```python
from build123d import *

# Parameters (mm, degrees)
SKETCH1_R           = 30
SKETCH1_R_2         = 7
BOSS_EXTRUDE1_DEPTH = 10
CUT_EXTRUDE1_DEPTH  = 161.838428244


with BuildPart() as part:
    # Sketch1 → Boss-Extrude1 (new, symmetric)
    with BuildSketch(Plane.XY):
        with BuildLine():
            Line((27.935473676, -25.760615491), (128.063755469, -9.084385863))
            ThreePointArc((128.063755469, -9.084385863), (155, 0), (128.063755469, 9.084385863))
            Line((128.063755469, 9.084385863), (27.935473676, 25.760615491))
            ThreePointArc((27.935473676, 25.760615491), (-38, 0), (27.935473676, -25.760615491))
        make_face()
        Circle(SKETCH1_R, mode=Mode.SUBTRACT)
        with Locations((140, 0)):
            Circle(SKETCH1_R_2, mode=Mode.SUBTRACT)
    extrude(amount=BOSS_EXTRUDE1_DEPTH, both=True)

    # Sketch2 → Cut-Extrude1 (cut, through all)
    with BuildSketch(Plane.XY.offset(10)):
        with BuildLine():
            Line((46.591424383, 15.557071672), (100.514303988, 6.576289156))
            ThreePointArc((100.514303988, 6.576289156), (106.085905266, 0), (100.514303988, -6.576289156))
            Line((100.514303988, -6.576289156), (46.591424383, -15.557071672))
            ThreePointArc((46.591424383, -15.557071672), (42.010455779, -13.921347897), (40.987646035, -9.165853617))
            ThreePointArc((40.987646035, -9.165853617), (42, 0), (40.987646035, 9.165853617))
            ThreePointArc((40.987646035, 9.165853617), (42.010455779, 13.921347897), (46.591424383, 15.557071672))
        make_face()
    extrude(amount=-CUT_EXTRUDE1_DEPTH, mode=Mode.SUBTRACT)


solid = part.part
```
Model file for the job. Use its own axes, mm. A direction names the side the tool comes from. Coordinates: 2 decimals unless noted, no trailing zeros. Write each loop counter-clockwise with the first axis right and the second up, starting at its lowest first coordinate (ties: lowest second). Pieces come first, ordered by that corner, then holes. Notation, with made-up numbers: (-33, 54.5) - (16, 54.5) arc R26 cw to (16, 78.5) - close; hole circle Ø4 at (-33, -9). An arc over 180 degrees is marked (long way). One line per item, written item: value. Start each with the question number.
1. Mould opens along Y. For faces 4 (the cylindrical face through (106.085, 0.131, 0.14)), 5 (the flat face through (77.3, -17.54, 0.14)), 6 (the flat face through (37, 0, 10)) say: released by +Y, released by -Y, zero draft, split by the parting line, or undercut.
2. Tool access for faces 1 (the flat face through (37, 0, -10)), 2 (the flat face through (78.701, 17.306, 0.14)), 3 (the cylindrical face through (42.058, -13.974, 0.14)): list every direction of +Z, -Z, +X, -X, +Y, -Y with a clear straight run to the whole face (end or side of a thin tool).
3. Slice it at A-A (y = 0). Write the cut outline in (x, z).
4. Slice it at D-D (y = 23.5). Write the cut outline in (x, z), plus the area to 3 significant figures.
5. Flat gauge pins, fed straight in: pin 1 (12 mm diameter, centred on y = -1.5, z = 6, fed in from +X); pin 2 (1 mm diameter, centred on x = 81, z = -1.5, fed in from +Y); pin 3 (1.5 mm diameter, centred on y = 16.5, z = 4, fed in from -X); pin 4 (1.5 mm diameter, centred on y = 25, z = -3, fed in from -X). Where does each tip first touch, or does it go through?
6. Slice it at B-B (x = 3.5). Write the cut outline in (y, z), plus the area to 3 significant figures.
7. Probe line 1 (Y direction, x = 0, z = -0.5); line 2 (Y direction, x = 140, z = -4.25); line 3 (Y direction, x = 129, z = 0). List the from-to ranges inside material, lowest first. Write a range as from..to.
8. Slice it at C-C (z = 4.75). Write the cut outline in (x, y) (3 decimals), plus the area to 3 significant figures.
Answers below:
1. face 4: undercut
1. face 5: released by -Y
1. face 6: zero draft
2. face 1: -Z, +X, -X, +Y, -Y
2. face 2: +Z, -Z, +Y
2. face 3: +Z, -Z
3. outline: (-38, -10) - (-30, -10) - (-30, 10) - (-38, 10) - close; (30, -10) - (42, -10) - (42, 10) - (30, 10) - close; (106.09, -10) - (133, -10) - (133, 10) - (106.09, 10) - close; (147, -10) - (155, -10) - (155, 10) - (147, 10) - close
4. outline: (-29.86, -10) - (-18.65, -10) - (-18.65, 10) - (-29.86, 10) - close; (18.65, -10) - (41.51, -10) - (41.51, 10) - (18.65, 10) - close
4. area: 681 mm^2
5. pin 1: stops at x = 155
5. pin 2: stops at y = 17.01
5. pin 3: stops at x = -34.58
5. pin 4: stops at x = -29.26
6. outline: (-37.84, -10) - (-29.8, -10) - (-29.8, 10) - (-37.84, 10) - close; (29.8, -10) - (37.84, -10) - (37.84, 10) - (29.8, 10) - close
6. area: 322 mm^2
7. line 1: y = -38..-30, 30..38
7. line 2: y = -15..-7, 7..15
7. line 3: y = -10.2..10.2
8. outline: (27.935, -25.761) - (128.064, -9.084) arc R15 ccw (long way) to (128.064, 9.084) - (27.935, 25.761) arc R38 ccw (long way) to start; hole circle Ø60 at (0, 0); hole (40.988, -9.166) arc R5 ccw to (46.591, -15.557) - (100.514, -6.576) arc R6.667 ccw to (100.514, 6.576) - (46.591, 15.557) arc R5 ccw to (40.988, 9.166) arc R42 cw to start; hole circle Ø14 at (140, 0)
8. area: 3,950 mm^2
